```python
from build123d import *

# Parameters (mm, degrees)
F1_DEPTH = 63.5
F0_W     = 25.4
F0_H     = 19.05
F2_DEPTH = 25.4
F3_DEPTH = 15.875
F5_R     = 6.35


with BuildPart() as f1:
    # F0 (on Front) → F1 (new body, symmetric)
    with BuildSketch(Plane.XZ):
        Polygon((-41.275, 9.525), (-41.275, -9.525), (41.275, -9.525), (41.275, 9.525), (22.225, 9.525), align=None)
    extrude(amount=F1_DEPTH, both=True)

    # F0 (on Front) → F2 (join, symmetric)
    with BuildSketch(Plane.XZ):
        with BuildLine():
            Line((22.225, 9.525), (41.275, 9.525))
            Line((41.275, 9.525), (41.275, 27.0002))
            ThreePointArc((41.275, 27.0002), (45.9246798487, 38.2255201513), (57.15, 42.8752))
            Line((57.15, 42.8752), (60.325, 42.8752))
            Line((60.325, 42.8752), (60.325, 61.9252))
            Line((60.325, 61.9252), (57.15, 61.9252))
            add(Edge.make_bspline(
                [(56.2394540171, 61.9133283476), (56.5421172975, 61.9177221898), (56.8456319814, 61.9216800485), (57.15, 61.9252)],
                knots=[111.0448358966, 111.0448358966, 111.0448358966, 111.0448358966, 111.5045361635, 111.5045361635, 111.5045361635, 111.5045361635], degree=3))
            ThreePointArc((56.2394540171, 61.9133283476), (32.1344404075, 51.371851632), (22.225, 27.0002))
            Line((22.225, 27.0002), (22.225, 9.525))
        make_face()
        with Locations((73.025, 52.4002)):
            Rectangle(F0_W, F0_H)
    extrude(amount=F2_DEPTH, both=True)

    # F0 (on Front) → F3 (join)
    with BuildSketch(Plane.XZ):
        with BuildLine():
            add(Edge.make_bspline(
                [(-41.275, 9.525), (-40.3026354638, 34.3505741686), (-16.871650594, 60.8519552711), (56.2394540171, 61.9133283476)],
                knots=[0, 0, 0, 0, 111.0448358966, 111.0448358966, 111.0448358966, 111.0448358966], degree=3))
            Line((-41.275, 9.525), (22.225, 9.525))
            Line((22.225, 9.525), (22.225, 27.0002))
            ThreePointArc((22.225, 27.0002), (32.1344404075, 51.371851632), (56.2394540171, 61.9133283476))
        make_face()
    extrude(amount=F3_DEPTH)

    # F0 (on Front) → F4 (revolve)
    with BuildSketch(Plane.XZ):
        Polygon((85.725, 66.675), (85.725, 61.9252), (85.725, 42.8752), (85.725, 38.1), (111.125, 38.1), (111.125, 66.675), align=None)
    revolve(axis=Axis((85.725, 0, 52.3875), (0, 0, 1)))

    # F5
    f5_edges = [f1.edges().sort_by_distance(p)[0] for p in [
        (41.275, -63.5, 0),
        (-41.275, -63.5, 0),
        (41.275, 63.5, 0),
        (-41.275, 63.5, 0),
    ]]
    fillet(f5_edges, radius=F5_R)


solid = f1.part
```
Check sheet for the modelled part. Datum: model origin and axes. Units: mm. A direction names the side the tool comes from. Give positions to 0.01 mm unless a question says otherwise; leave off trailing zeros. Loops run counter-clockwise (first coordinate to the right, second up) from the corner with the lowest first, then second, coordinate; pieces in that order, holes last. Notation, with made-up numbers: M 8.5,15 L 14.5,15 A31 cw 14.5,48 Z; hole C 15.25,70 d4. An arc over 180 degrees is marked long. Answer in a Markdown table with one row per item.
1) Mould release check, pull along X, two halves, no side actions. Record for faces 1 (the face through (32.4, -20.7, 51.64)), 2 (the face through (86, 0, 38.1)), 3 (the face through (45.8, -0.4, 38.1)): released by +X, released by -X, zero draft, split by the parting line, or undercut.
Solutions:
| item | result |
|---|---|
| face 1 | released by -X |
| face 2 | zero draft |
| face 3 | undercut |
2) Thickness scan on line 1 (X direction, y = -34.5, z = -5.5) (3 decimals); line 2 (Z direction, x = -33.5, y = 24.5) (3 decimals); line 3 (X direction, y = 20.5, z = 14) (3 decimals). Record the ranges inside material, lowest first.
Solutions:
| item | result |
|---|---|
| line 1 | x = -41.275 to 41.275 |
| line 2 | z = -9.525 to 9.525 |
| line 3 | x = 22.225 to 41.275 |
3) Cross-section at A-A (z = 5.5). Enter the section's corners in (x, y) (3 decimals).
Solutions:
| item | result |
|---|---|
| outline | M -41.275,-57.15 A6.35 ccw -34.925,-63.5 L 34.925,-63.5 A6.35 ccw 41.275,-57.15 L 41.275,57.15 A6.35 ccw 34.925,63.5 L -34.925,63.5 A6.35 ccw -41.275,57.15 Z |
4) Cross-section at D-D (x = 99). Enter the section's corners in (y, z) (3 decimals), plus the area to 3 significant figures.
Solutions:
| item | result |
|---|---|
| outline | M -21.655,38.1 L 21.655,38.1 L 21.655,66.675 L -21.655,66.675 Z |
| area | 1,240 mm^2 |
5) Cross-section at B-B (y = 49.5). Enter the section's corners in (x, z) (3 decimals).
Solutions:
| item | result |
|---|---|
| outline | M -41.275,-9.525 L 41.275,-9.525 L 41.275,9.525 L -41.275,9.525 Z |
6) Tool access check on faces 4 (the face through (32.4, 12.52, 51.64)), 5 (the face through (60, -2, 61.925)), 6 (the face through (41.275, -1, 4)), 7 (the face through (60, 2, 42.875)), 8 (the face through (46, -25.4, 42)). Record the directions out of +Z, -Z, +X, -X, +Y, -Y that give a thin tool (end or side, any length) a straight path to the whole face; none if there is none.
Solutions:
| item | result |
|---|---|
| face 4 | +Z, -X, +Y |
| face 5 | +Z, -X |
| face 6 | -Z, +X, +Y, -Y |
| face 7 | -Z |
| face 8 | +Z, +X, -X, -Y |
7) Depth check by flat-ended pin: pin 1 (6 mm diameter, centred on x = 26, y = -38, fed in from +Z) (3 decimals); pin 2 (15.5 mm diameter, centred on x = 24.5, z = 29.5, fed in from -Y); pin 3 (11 mm diameter, centred on y = -23.5, z = 3, fed in from +X) (3 decimals). Enter the tip coordinate at first touch or a pass-through.
Solutions:
| item | result |
|---|---|
| pin 1 | stops at z = 9.525 |
| pin 2 | stops at y = -25.4 |
| pin 3 | stops at x = 41.275 |
8) Cross-section at C-C (x = 77). Enter the section's corners in (y, z) (3 decimals).
Solutions:
| item | result |
|---|---|
| outline | M -25.4,42.875 L -23.854,42.875 L -23.854,38.1 L 23.854,38.1 L 23.854,42.875 L 25.4,42.875 L 25.4,61.925 L 23.854,61.925 L 23.854,66.675 L -23.854,66.675 L -23.854,61.925 L -25.4,61.925 Z |
